For this review, take the finished solid that the model builds, in its own axes (mm). Face numbers are marked on the shaded views. Coordinates: 2 decimals unless noted, no trailing zeros. Loops run counter-clockwise (first coordinate to the right, second up) from the corner with the lowest first, then second, coordinate; pieces in that order, holes last. Notation, with made-up numbers: (26, 31.25) - (62, 31.25) arc R13 ccw to (62, 42.25) - close; hole circle Ø5 at (63.25, 0). An arc over 180 degrees is marked (long way). Answer as a JSON object with one key per item and string values. Group by question number.
Item 1: Mouldability with a two-part tool opening along X and no side actions: class the marked faces 1, 2 and 3 as released by +X, released by -X, zero draft, split by the parting line, or undercut.
Item 2: We need section A-A (z = 22). Give the boundary of the cut face in (x, y), then the cut area to 3 significant figures.
Item 3: We need section B-B (y = 0). Give the boundary of the cut face in (x, z), then the cut area to 3 significant figures.
Item 4: Clearance check with flat-ended pins moving along their axes: pin 1 (1.7 mm diameter, centred on y = -1, z = 20, fed in from +X); pin 2 (6 mm diameter, centred on x = 4.5, z = 40.5, fed in from +Y); pin 3 (1.1 mm diameter, centred on x = -4, y = 2.5, fed in from -Z); pin 4 (2 mm diameter, centred on x = -2.5, y = -2.5, fed in from +Z). State where each tip first meets the part, or that it passes through.
Item 5: To check wall thickness, follow line 1 (X direction, y = -0.25, z = 4.5); line 2 (X direction, y = 1.5, z = 40.5); line 3 (Y direction, x = -2.25, z = 46). State the ranges of each line that lie inside material, in increasing order.
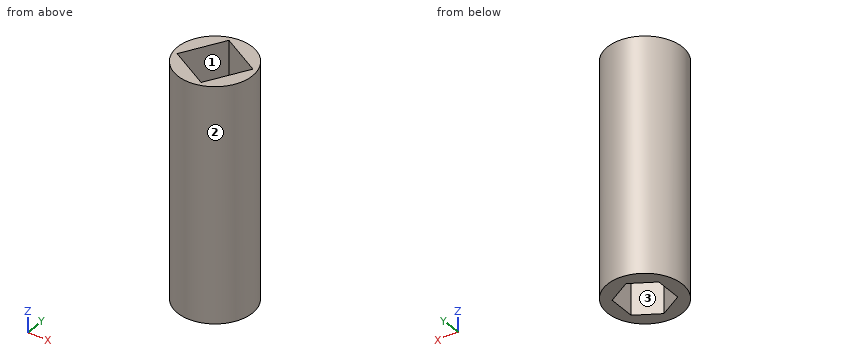
from build123d import *

# Parameters (mm, degrees)
SKETCH_R     = 8
PAD_DEPTH    = 40
SKETCH001_R  = 8
PAD001_DEPTH = 10


with BuildPart() as part:
    # Sketch → Pad (new body)
    with BuildSketch(Plane.XY):
        Circle(SKETCH_R)
        Polygon((5, -2.886751), (5, 2.886751), (0, 5.773503), (-5, 2.886751), (-5, -2.886751), (0, -5.773503), align=None, mode=Mode.SUBTRACT)
    extrude(amount=PAD_DEPTH)

    # Sketch001 → Pad001 (join)
    with BuildSketch(Plane.XY.offset(40)):
        Circle(SKETCH001_R)
        Polygon((-1.830127, 6.830127), (-6.830127, -1.830127), (1.830127, -6.830127), (6.830127, 1.830127), align=None, mode=Mode.SUBTRACT)
    extrude(amount=PAD001_DEPTH)


solid = part.part
Check sheet entries:
{
 "1": {"face 1": "undercut", "face 2": "split by the parting line", "face 3": "undercut"},
 "2": {"outline": "circle Ø16 at (0, 0); hole (-5, -2.89) - (0, -5.77) - (5, -2.89) - (5, 2.89) - (0, 5.77) - (-5, 2.89) - close", "area": "114 mm2"},
 "3": {"outline": "(-8, 0) - (-5, 0) - (-5, 40) - (-5.77, 40) - (-5.77, 50) - (-8, 50) - close; (5, 0) - (8, 0) - (8, 50) - (5.77, 50) - (5.77, 40) - (5, 40) - close", "area": "285 mm2"},
 "4": {"pin 1": "stops at x = 8", "pin 2": "stops at y = 7.86", "pin 3": "stops at z = 40", "pin 4": "passes through"},
 "5": {"line 1": "x = -8 to -5, 5 to 8", "line 2": "x = -7.86 to -4.91, 6.64 to 7.86", "line 3": "y = -7.68 to -4.47, 6.1 to 7.68"}
}
